```python
from build123d import *

# Parameters (mm, degrees)
SKETCH086_R   = 3
SKETCH086_R_2 = 2


with BuildPart() as part:
    # AdditivePipe002: sweep along a path in Sketch085
    with BuildLine(Plane.YZ) as additivepipe002_path:
        Line((0, 0), (8.080041, 0))
        ThreePointArc((8.080041, 0), (15.441707, 6.195646), (10.594056, 14.50711))
        ThreePointArc((10.594056, 14.50711), (2.14173, 20.933751), (-1.066078, 31.055682))
        Line((-1.066078, 31.055682), (-1.066078, 57.808475))
    # Sketch086 → AdditivePipe002 (sweep)
    with BuildSketch(Plane.XZ):
        Circle(SKETCH086_R)
        Circle(SKETCH086_R_2, mode=Mode.SUBTRACT)
    sweep(path=additivepipe002_path.line, is_frenet=True)


solid = part.part
```
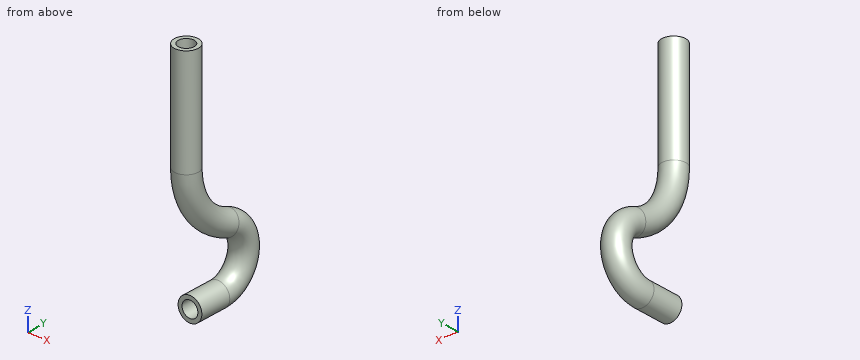
Geometry check sheet. Reference: the model listing, model coordinates, mm. Round coordinates to 2 decimals unless told otherwise and drop trailing zeros. Return JSON: item names as keys, results as strings. Group by question number.
(1) Section check A-A, the plane y = 10. Give the number of separate pieces and of enclosed holes in the cut face, and give its area (3 significant figures).
(2) Go/stop test with flat-tipped pins: pin 1 (1.8 mm diameter, centred on x = -0.5, z = 0, fed in from -Y); pin 2 (2.5 mm diameter, centred on x = 0, z = 0, fed in from -Y); pin 3 (1.5 mm diameter, centred on x = -2, z = 9.5, fed in from +Y). Record where each tip stops, or that it passes through.
(3) Scan lines: line 1 along Z through (x, y) = (0, 5.5); line 2 along Z through (x, y) = (0.5, 8.5); line 3 along Y through (x, z) = (0.75, 29.5). Record each from-to range of solid material in increasing order. Write a range as [from, to].
Data:
{
 "1": {"separate pieces": "2", "enclosed holes": "2", "area": "33.4 mm²"},
 "2": {"pin 1": "y = 12.22", "pin 2": "y = 11.77", "pin 3": "y = 18.1"},
 "3": {"line 1": "[-3, -2], [2, 3], [13.67, 14.87], [20.04, 21.5]", "line 2": "[-2.95, -1.93], [1.95, 2.98], [12.15, 13.26], [17.62, 18.83]", "line 3": "[-3.91, -2.86], [0.87, 1.92]"}
}
